Geometry check sheet. Reference: the model listing, model coordinates, mm. Face numbers are marked on the shaded views. A direction names the side the tool comes from. Coordinates: 2 decimals unless noted, no trailing zeros. Write each loop counter-clockwise with the first axis right and the second up, starting at its lowest first coordinate (ties: lowest second). Pieces come first, ordered by that corner, then holes. Notation, with made-up numbers: M 75.25,89 L 127.25,89 A12 cw 127.25,101 Z; hole C 6,72 d10. An arc over 180 degrees is marked long. Write each question's results on one line, items separated by ' | '.
```python
from build123d import *

# Parameters (mm, degrees)
BOSS_EXTRUDE1_DEPTH = 100
SKETCH2_R           = 4
CUT_EXTRUDE1_DEPTH  = 208.665596573
SKETCH3_R           = 4
CUT_EXTRUDE2_DEPTH  = 207.518764281
SKETCH4_W           = 30
SKETCH4_H           = 180
BOSS_EXTRUDE2_DEPTH = 5
SKETCH5_R           = 4.915
BOSS_EXTRUDE3_DEPTH = 30
SKETCH6_W           = 24.13
SKETCH6_H           = 109.462544294
CUT_EXTRUDE3_DEPTH  = 256.049014897


with BuildPart() as part:
    # Sketch1 → Boss-Extrude1 (new body)
    with BuildSketch(Plane.XY):
        Polygon((0, 50), (5, 50), (5, 5), (170, 5), (170, 50), (175, 50), (175, 0), (0, 0), align=None)
    extrude(amount=BOSS_EXTRUDE1_DEPTH)

    # Sketch2 → Cut-Extrude1 (cut, through all)
    with BuildSketch(Plane.ZY):
        with Locations((80, 30)):
            Circle(SKETCH2_R)
        with BuildLine():
            Line((100, 30), (100, 5))
            Line((100, 5), (131.663980624, 33.697237635))
            Line((131.663980624, 33.697237635), (100, 64.741873333))
            Line((100, 64.741873333), (-14.790865649, 55.926144723))
            Line((-14.790865649, 55.926144723), (0, 5))
            Line((0, 5), (69.651665268, 47.114671141))
            ThreePointArc((69.651665268, 47.114671141), (89.824288915, 47.420773442), (100, 30))
        make_face()
    extrude(amount=-CUT_EXTRUDE1_DEPTH, mode=Mode.SUBTRACT)

    # Sketch3 → Cut-Extrude2 (cut, through all)
    with BuildSketch(Plane(origin=(0, 5, 0), x_dir=(1, 0, 0), z_dir=(0, 1, 0))):
        with Locations(Location((20, -15, 0), (0, 0, 270))):
            Circle(SKETCH3_R)
        with Locations(Location((155, -15, 0), (0, 0, 270))):
            Circle(SKETCH3_R)
        with Locations(Location((155, -85, 0), (0, 0, 270))):
            Circle(SKETCH3_R)
        with Locations(Location((20, -85, 0), (0, 0, 270))):
            Circle(SKETCH3_R)
    extrude(amount=-CUT_EXTRUDE2_DEPTH, mode=Mode.SUBTRACT)

    # Sketch4 → Boss-Extrude2 (add)
    with BuildSketch(Plane(origin=(0, 5, 0), x_dir=(1, 0, 0), z_dir=(0, 1, 0))):
        with Locations((20, 90)):
            Rectangle(SKETCH4_W, SKETCH4_H)
    extrude(amount=-BOSS_EXTRUDE2_DEPTH)

    # Sketch5 → Boss-Extrude3 (add)
    with BuildSketch(Plane.ZY.offset(-5)):
        with BuildLine():
            Line((-180, 18), (-180, 5))
            Line((-180, 5), (-154.6, 5))
            Line((-154.6, 5), (-154.6, 18))
            ThreePointArc((-154.6, 18), (-167.3, 30.7), (-180, 18))
        make_face()
        with Locations((-167.3, 18)):
            Circle(SKETCH5_R, mode=Mode.SUBTRACT)
    extrude(amount=-BOSS_EXTRUDE3_DEPTH)

    # Sketch6 → Cut-Extrude3 (cut, through all)
    with BuildSketch(Plane(origin=(0, 5, 0), x_dir=(1, 0, 0), z_dir=(0, 1, 0))):
        with Locations((20, 162.88766727)):
            Rectangle(SKETCH6_W, SKETCH6_H)
    extrude(amount=CUT_EXTRUDE3_DEPTH, mode=Mode.SUBTRACT)


solid = part.part
```
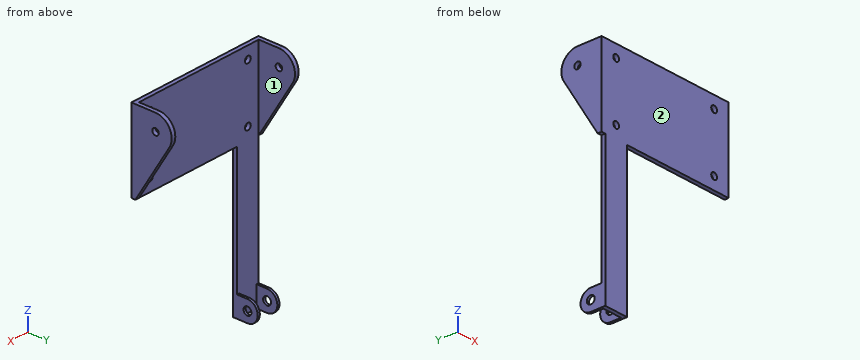
Q1. Sectioned sample at B-B on y = 37. Record the cut outline in (x, z) (3 decimals).
Geometry check:
outline: M 0,52.923 L 5,52.923 L 5,98.735 L 0,98.735 Z; M 170,52.923 L 175,52.923 L 175,98.735 L 170,98.735 Z
Q2. Depth check by flat-ended pin: P1, Ø4, axis at x = 73, y = 3, coming from the -Z side; P2, Ø0.9, axis at x = 6.5, y = 10, coming from the +Z side; P3, Ø13, axis at x = 155, z = 85, coming from the +Y side. Enter the tip coordinate at first touch or a pass-through.
Geometry check:
P1: stops at z = 0 | P2: stops at z = -154.6 | P3: stops at y = 5
Q3. Sectioned sample at D-D on z = 34. Record the cut outline in (x, y), and give its area (3 significant figures).
Geometry check:
outline: M 0,0 L 175,0 L 175,25.56 L 170,25.56 L 170,5 L 5,5 L 5,25.56 L 0,25.56 Z | area: 1,080 mm2
Q4. Access from +Z, -Z, +X, -X, +Y, -Y to the whole of each face (thin tool, end or side, straight path). Record for the marked faces 1 and 2.
Geometry check:
face 1: +Z, +Y | face 2: +Z, -Z, +X, -X, -Y
Q5. Sectioned sample at C-C on y = 8. Record the cut outline in (x, z) (3 decimals), and give its area (3 significant figures).
Geometry check:
outline: M 0,4.962 L 5,4.962 L 5,100 L 0,100 Z; M 5,-180 L 7.935,-180 L 7.935,-154.6 L 5,-154.6 Z; M 32.065,-180 L 35,-180 L 35,-154.6 L 32.065,-154.6 Z; M 170,4.962 L 175,4.962 L 175,100 L 170,100 Z | area: 1,100 mm2
Q6. Scan lines: probe 1 along X at (y, z) = (1.6, 15); probe 2 along Y at (x, z) = (2, 80); probe 3 along X at (y, z) = (13, 58). Record each from-to range of solid material in increasing order.
Geometry check:
probe 1: x = 0 to 16, 24 to 151, 159 to 175 | probe 2: y = 0 to 26, 34 to 50 | probe 3: x = 0 to 5, 170 to 175
Q7. Sectioned sample at A-A on z = -167.3. Record the cut outline in (x, y) (3 decimals).
Geometry check:
outline: M 5,0 L 35,0 L 35,13.085 L 32.065,13.085 L 32.065,5 L 7.935,5 L 7.935,13.085 L 5,13.085 Z; M 5,22.915 L 7.935,22.915 L 7.935,30.7 L 5,30.7 Z; M 32.065,22.915 L 35,22.915 L 35,30.7 L 32.065,30.7 Z
